```python
from build123d import *

# Parameters (mm, degrees)
SKETCH_1_W          = 15
SKETCH_1_H          = 15
SKETCH_1_W_2        = 13
SKETCH_1_H_2        = 13
EXTRUDE_1_DEPTH     = 125
CUT_EXTRUDE_1_REACH = 128.12
SKETCH_2_R          = 1.575
CUT_EXTRUDE_2_REACH = 128.12
SKETCH_3_R          = 1.6


with BuildPart() as part:
    # 草图1 → 凸台-拉伸1 (new body)
    with BuildSketch(Plane(origin=(0, 0, 0), x_dir=(1, 0, 0), z_dir=(0, 1, 0))):
        Rectangle(SKETCH_1_W, SKETCH_1_H)
        Rectangle(SKETCH_1_W_2, SKETCH_1_H_2, mode=Mode.SUBTRACT)
    extrude(amount=EXTRUDE_1_DEPTH)

    # 切除-拉伸1: up to this face of the body (flat: up to its plane)
    cut_extrude_1_end = Plane(part.part.faces().sort_by_distance((0, 62.5, -7.5))[0])
    # 草图2 → 切除-拉伸1 (cut, up to the picked face)
    with BuildSketch(Plane.XY.offset(7.5), mode=Mode.PRIVATE) as cut_extrude_1_sk1:
        with Locations((-3.75, 67.5)):
            Circle(SKETCH_2_R)
    cut_extrude_1_tool1 = split(extrude(cut_extrude_1_sk1.sketch, amount=-CUT_EXTRUDE_1_REACH, mode=Mode.PRIVATE), bisect_by=cut_extrude_1_end, keep=Keep.BOTH, mode=Mode.PRIVATE)
    # 草图2 → 切除-拉伸1 (cut, up to the picked face)
    with BuildSketch(Plane.XY.offset(7.5), mode=Mode.PRIVATE) as cut_extrude_1_sk2:
        with Locations((3.75, 67.5)):
            Circle(SKETCH_2_R)
    cut_extrude_1_tool2 = split(extrude(cut_extrude_1_sk2.sketch, amount=-CUT_EXTRUDE_1_REACH, mode=Mode.PRIVATE), bisect_by=cut_extrude_1_end, keep=Keep.BOTH, mode=Mode.PRIVATE)
    # 草图2 → 切除-拉伸1 (cut, up to the picked face)
    with BuildSketch(Plane.XY.offset(7.5), mode=Mode.PRIVATE) as cut_extrude_1_sk3:
        with Locations((-3.75, 57.5)):
            Circle(SKETCH_2_R)
    cut_extrude_1_tool3 = split(extrude(cut_extrude_1_sk3.sketch, amount=-CUT_EXTRUDE_1_REACH, mode=Mode.PRIVATE), bisect_by=cut_extrude_1_end, keep=Keep.BOTH, mode=Mode.PRIVATE)
    # 草图2 → 切除-拉伸1 (cut, up to the picked face)
    with BuildSketch(Plane.XY.offset(7.5), mode=Mode.PRIVATE) as cut_extrude_1_sk4:
        with Locations((3.75, 57.5)):
            Circle(SKETCH_2_R)
    cut_extrude_1_tool4 = split(extrude(cut_extrude_1_sk4.sketch, amount=-CUT_EXTRUDE_1_REACH, mode=Mode.PRIVATE), bisect_by=cut_extrude_1_end, keep=Keep.BOTH, mode=Mode.PRIVATE)
    # 草图2 → 切除-拉伸1 (cut, up to the picked face)
    with BuildSketch(Plane.XY.offset(7.5), mode=Mode.PRIVATE) as cut_extrude_1_sk5:
        with Locations((3.75, 120)):
            Circle(SKETCH_2_R)
    cut_extrude_1_tool5 = split(extrude(cut_extrude_1_sk5.sketch, amount=-CUT_EXTRUDE_1_REACH, mode=Mode.PRIVATE), bisect_by=cut_extrude_1_end, keep=Keep.BOTH, mode=Mode.PRIVATE)
    # 草图2 → 切除-拉伸1 (cut, up to the picked face)
    with BuildSketch(Plane.XY.offset(7.5), mode=Mode.PRIVATE) as cut_extrude_1_sk6:
        with Locations((-3.75, 120)):
            Circle(SKETCH_2_R)
    cut_extrude_1_tool6 = split(extrude(cut_extrude_1_sk6.sketch, amount=-CUT_EXTRUDE_1_REACH, mode=Mode.PRIVATE), bisect_by=cut_extrude_1_end, keep=Keep.BOTH, mode=Mode.PRIVATE)
    # 草图2 → 切除-拉伸1 (cut, up to the picked face)
    with BuildSketch(Plane.XY.offset(7.5), mode=Mode.PRIVATE) as cut_extrude_1_sk7:
        with Locations((-3.75, 110)):
            Circle(SKETCH_2_R)
    cut_extrude_1_tool7 = split(extrude(cut_extrude_1_sk7.sketch, amount=-CUT_EXTRUDE_1_REACH, mode=Mode.PRIVATE), bisect_by=cut_extrude_1_end, keep=Keep.BOTH, mode=Mode.PRIVATE)
    # 草图2 → 切除-拉伸1 (cut, up to the picked face)
    with BuildSketch(Plane.XY.offset(7.5), mode=Mode.PRIVATE) as cut_extrude_1_sk8:
        with Locations((3.75, 110)):
            Circle(SKETCH_2_R)
    cut_extrude_1_tool8 = split(extrude(cut_extrude_1_sk8.sketch, amount=-CUT_EXTRUDE_1_REACH, mode=Mode.PRIVATE), bisect_by=cut_extrude_1_end, keep=Keep.BOTH, mode=Mode.PRIVATE)
    # 草图2 → 切除-拉伸1 (cut, up to the picked face)
    with BuildSketch(Plane.XY.offset(7.5), mode=Mode.PRIVATE) as cut_extrude_1_sk9:
        with Locations((3.75, 15)):
            Circle(SKETCH_2_R)
    cut_extrude_1_tool9 = split(extrude(cut_extrude_1_sk9.sketch, amount=-CUT_EXTRUDE_1_REACH, mode=Mode.PRIVATE), bisect_by=cut_extrude_1_end, keep=Keep.BOTH, mode=Mode.PRIVATE)
    # 草图2 → 切除-拉伸1 (cut, up to the picked face)
    with BuildSketch(Plane.XY.offset(7.5), mode=Mode.PRIVATE) as cut_extrude_1_sk10:
        with Locations((-3.75, 15)):
            Circle(SKETCH_2_R)
    cut_extrude_1_tool10 = split(extrude(cut_extrude_1_sk10.sketch, amount=-CUT_EXTRUDE_1_REACH, mode=Mode.PRIVATE), bisect_by=cut_extrude_1_end, keep=Keep.BOTH, mode=Mode.PRIVATE)
    # 草图2 → 切除-拉伸1 (cut, up to the picked face)
    with BuildSketch(Plane.XY.offset(7.5), mode=Mode.PRIVATE) as cut_extrude_1_sk11:
        with Locations((-3.75, 5)):
            Circle(SKETCH_2_R)
    cut_extrude_1_tool11 = split(extrude(cut_extrude_1_sk11.sketch, amount=-CUT_EXTRUDE_1_REACH, mode=Mode.PRIVATE), bisect_by=cut_extrude_1_end, keep=Keep.BOTH, mode=Mode.PRIVATE)
    # 草图2 → 切除-拉伸1 (cut, up to the picked face)
    with BuildSketch(Plane.XY.offset(7.5), mode=Mode.PRIVATE) as cut_extrude_1_sk12:
        with Locations((3.75, 5)):
            Circle(SKETCH_2_R)
    cut_extrude_1_tool12 = split(extrude(cut_extrude_1_sk12.sketch, amount=-CUT_EXTRUDE_1_REACH, mode=Mode.PRIVATE), bisect_by=cut_extrude_1_end, keep=Keep.BOTH, mode=Mode.PRIVATE)
    add(cut_extrude_1_tool1.solids().sort_by(Axis((-3.75, 67.5, 7.5), (0, 0, -1)))[0], mode=Mode.SUBTRACT)
    add(cut_extrude_1_tool2.solids().sort_by(Axis((3.75, 67.5, 7.5), (0, 0, -1)))[0], mode=Mode.SUBTRACT)
    add(cut_extrude_1_tool3.solids().sort_by(Axis((-3.75, 57.5, 7.5), (0, 0, -1)))[0], mode=Mode.SUBTRACT)
    add(cut_extrude_1_tool4.solids().sort_by(Axis((3.75, 57.5, 7.5), (0, 0, -1)))[0], mode=Mode.SUBTRACT)
    add(cut_extrude_1_tool5.solids().sort_by(Axis((3.75, 120, 7.5), (0, 0, -1)))[0], mode=Mode.SUBTRACT)
    add(cut_extrude_1_tool6.solids().sort_by(Axis((-3.75, 120, 7.5), (0, 0, -1)))[0], mode=Mode.SUBTRACT)
    add(cut_extrude_1_tool7.solids().sort_by(Axis((-3.75, 110, 7.5), (0, 0, -1)))[0], mode=Mode.SUBTRACT)
    add(cut_extrude_1_tool8.solids().sort_by(Axis((3.75, 110, 7.5), (0, 0, -1)))[0], mode=Mode.SUBTRACT)
    add(cut_extrude_1_tool9.solids().sort_by(Axis((3.75, 15, 7.5), (0, 0, -1)))[0], mode=Mode.SUBTRACT)
    add(cut_extrude_1_tool10.solids().sort_by(Axis((-3.75, 15, 7.5), (0, 0, -1)))[0], mode=Mode.SUBTRACT)
    add(cut_extrude_1_tool11.solids().sort_by(Axis((-3.75, 5, 7.5), (0, 0, -1)))[0], mode=Mode.SUBTRACT)
    add(cut_extrude_1_tool12.solids().sort_by(Axis((3.75, 5, 7.5), (0, 0, -1)))[0], mode=Mode.SUBTRACT)

    # 切除-拉伸2: up to this face of the body (flat: up to its plane)
    cut_extrude_2_end = Plane(part.part.faces().sort_by_distance((7.5, 62.5, 0))[0])
    # 草图3 → 切除-拉伸2 (cut, up to the picked face)
    with BuildSketch(Plane.ZY.offset(7.5), mode=Mode.PRIVATE) as cut_extrude_2_sk1:
        with Locations((-3.75, 87.5)):
            Circle(SKETCH_3_R)
    cut_extrude_2_tool1 = split(extrude(cut_extrude_2_sk1.sketch, amount=-CUT_EXTRUDE_2_REACH, mode=Mode.PRIVATE), bisect_by=cut_extrude_2_end, keep=Keep.BOTH, mode=Mode.PRIVATE)
    # 草图3 → 切除-拉伸2 (cut, up to the picked face)
    with BuildSketch(Plane.ZY.offset(7.5), mode=Mode.PRIVATE) as cut_extrude_2_sk2:
        with Locations((3.75, 87.5)):
            Circle(SKETCH_3_R)
    cut_extrude_2_tool2 = split(extrude(cut_extrude_2_sk2.sketch, amount=-CUT_EXTRUDE_2_REACH, mode=Mode.PRIVATE), bisect_by=cut_extrude_2_end, keep=Keep.BOTH, mode=Mode.PRIVATE)
    # 草图3 → 切除-拉伸2 (cut, up to the picked face)
    with BuildSketch(Plane.ZY.offset(7.5), mode=Mode.PRIVATE) as cut_extrude_2_sk3:
        with Locations((-3.75, 77.5)):
            Circle(SKETCH_3_R)
    cut_extrude_2_tool3 = split(extrude(cut_extrude_2_sk3.sketch, amount=-CUT_EXTRUDE_2_REACH, mode=Mode.PRIVATE), bisect_by=cut_extrude_2_end, keep=Keep.BOTH, mode=Mode.PRIVATE)
    # 草图3 → 切除-拉伸2 (cut, up to the picked face)
    with BuildSketch(Plane.ZY.offset(7.5), mode=Mode.PRIVATE) as cut_extrude_2_sk4:
        with Locations((3.75, 77.5)):
            Circle(SKETCH_3_R)
    cut_extrude_2_tool4 = split(extrude(cut_extrude_2_sk4.sketch, amount=-CUT_EXTRUDE_2_REACH, mode=Mode.PRIVATE), bisect_by=cut_extrude_2_end, keep=Keep.BOTH, mode=Mode.PRIVATE)
    # 草图3 → 切除-拉伸2 (cut, up to the picked face)
    with BuildSketch(Plane.ZY.offset(7.5), mode=Mode.PRIVATE) as cut_extrude_2_sk5:
        with Locations((3.75, 47.5)):
            Circle(SKETCH_3_R)
    cut_extrude_2_tool5 = split(extrude(cut_extrude_2_sk5.sketch, amount=-CUT_EXTRUDE_2_REACH, mode=Mode.PRIVATE), bisect_by=cut_extrude_2_end, keep=Keep.BOTH, mode=Mode.PRIVATE)
    # 草图3 → 切除-拉伸2 (cut, up to the picked face)
    with BuildSketch(Plane.ZY.offset(7.5), mode=Mode.PRIVATE) as cut_extrude_2_sk6:
        with Locations((-3.75, 47.5)):
            Circle(SKETCH_3_R)
    cut_extrude_2_tool6 = split(extrude(cut_extrude_2_sk6.sketch, amount=-CUT_EXTRUDE_2_REACH, mode=Mode.PRIVATE), bisect_by=cut_extrude_2_end, keep=Keep.BOTH, mode=Mode.PRIVATE)
    # 草图3 → 切除-拉伸2 (cut, up to the picked face)
    with BuildSketch(Plane.ZY.offset(7.5), mode=Mode.PRIVATE) as cut_extrude_2_sk7:
        with Locations((3.75, 37.5)):
            Circle(SKETCH_3_R)
    cut_extrude_2_tool7 = split(extrude(cut_extrude_2_sk7.sketch, amount=-CUT_EXTRUDE_2_REACH, mode=Mode.PRIVATE), bisect_by=cut_extrude_2_end, keep=Keep.BOTH, mode=Mode.PRIVATE)
    # 草图3 → 切除-拉伸2 (cut, up to the picked face)
    with BuildSketch(Plane.ZY.offset(7.5), mode=Mode.PRIVATE) as cut_extrude_2_sk8:
        with Locations((-3.75, 37.5)):
            Circle(SKETCH_3_R)
    cut_extrude_2_tool8 = split(extrude(cut_extrude_2_sk8.sketch, amount=-CUT_EXTRUDE_2_REACH, mode=Mode.PRIVATE), bisect_by=cut_extrude_2_end, keep=Keep.BOTH, mode=Mode.PRIVATE)
    add(cut_extrude_2_tool1.solids().sort_by(Axis((-7.5, 87.5, -3.75), (1, 0, 0)))[0], mode=Mode.SUBTRACT)
    add(cut_extrude_2_tool2.solids().sort_by(Axis((-7.5, 87.5, 3.75), (1, 0, 0)))[0], mode=Mode.SUBTRACT)
    add(cut_extrude_2_tool3.solids().sort_by(Axis((-7.5, 77.5, -3.75), (1, 0, 0)))[0], mode=Mode.SUBTRACT)
    add(cut_extrude_2_tool4.solids().sort_by(Axis((-7.5, 77.5, 3.75), (1, 0, 0)))[0], mode=Mode.SUBTRACT)
    add(cut_extrude_2_tool5.solids().sort_by(Axis((-7.5, 47.5, 3.75), (1, 0, 0)))[0], mode=Mode.SUBTRACT)
    add(cut_extrude_2_tool6.solids().sort_by(Axis((-7.5, 47.5, -3.75), (1, 0, 0)))[0], mode=Mode.SUBTRACT)
    add(cut_extrude_2_tool7.solids().sort_by(Axis((-7.5, 37.5, 3.75), (1, 0, 0)))[0], mode=Mode.SUBTRACT)
    add(cut_extrude_2_tool8.solids().sort_by(Axis((-7.5, 37.5, -3.75), (1, 0, 0)))[0], mode=Mode.SUBTRACT)


solid = part.part
```
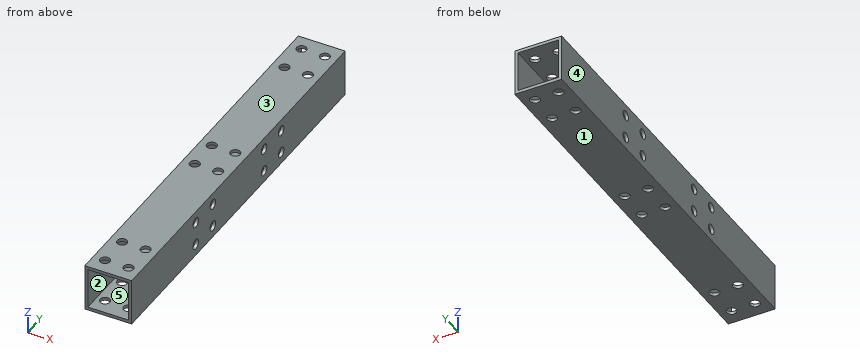
CAD build for the part. Positions are in the model's coordinates, mm. Face numbers are marked on the shaded views. A direction names the side the tool comes from. Give positions to 0.01 mm unless a question says otherwise; leave off trailing zeros. Loops run counter-clockwise (first coordinate to the right, second up) from the corner with the lowest first, then second, coordinate; pieces in that order, holes last. Notation, with made-up numbers: (-12.75, 34) - (-2.75, 34) arc R17 cw to (-2.75, 44) - close; hole circle Ø11 at (40, -10). An arc over 180 degrees is marked (long way). Put each result on its own line as item: value.
Q1. Flat gauge pin, fed straight in: pin 1 (2.5 mm diameter, centred on y = 87.5, z = 3.75, fed in from -X). Where does the tip first touch, or does it go through?
Filled in:
pin 1: passes through
Q2. Tool access for the marked faces 1 and 2: list every direction of +Z, -Z, +X, -X, +Y, -Y with a clear straight run to the whole face (end or side of a thin tool).
Filled in:
face 1: -Z, +X, -X, +Y, -Y
face 2: +Y, -Y
Q3. Slice it at D-D (x = -3.75). Give the number of separate pieces and of enclosed holes in the cut face, plus the area to 3 significant figures.
Filled in:
separate pieces: 14
enclosed holes: 0
area: 212 mm²
Q4. Slice it at C-C (y = 15). Give the cut face in (x, z) (3 decimals), plus the area to 3 significant figures.
Filled in:
outline: (-7.5, -7.5) - (-5.325, -7.5) - (-5.325, -6.5) - (-6.5, -6.5) - (-6.5, 6.5) - (-5.325, 6.5) - (-5.325, 7.5) - (-7.5, 7.5) - close; (-2.175, -7.5) - (2.175, -7.5) - (2.175, -6.5) - (-2.175, -6.5) - close; (-2.175, 6.5) - (2.175, 6.5) - (2.175, 7.5) - (-2.175, 7.5) - close; (5.325, -7.5) - (7.5, -7.5) - (7.5, 7.5) - (5.325, 7.5) - (5.325, 6.5) - (6.5, 6.5) - (6.5, -6.5) - (5.325, -6.5) - close
area: 43.4 mm²
Q5. Mould opens along X. For the marked faces 3, 4 and 5 say: pulls with the +X half, pulls with the -X half, needs draft (parallel to the pull), parting line crosses it, or undercut.
Filled in:
face 3: needs draft
face 4: pulls with the -X half
face 5: undercut
Q6. Slice it at B-B (z = 1). Give the cut face in (x, y).
Filled in:
outline: (-7.5, 0) - (-6.5, 0) - (-6.5, 125) - (-7.5, 125) - close; (6.5, 0) - (7.5, 0) - (7.5, 125) - (6.5, 125) - close
Q7. Slice it at A-A (y = 52). Give the cut face in (x, z).
Filled in:
outline: (-7.5, -7.5) - (7.5, -7.5) - (7.5, 7.5) - (-7.5, 7.5) - close; hole (-6.5, -6.5) - (6.5, -6.5) - (6.5, 6.5) - (-6.5, 6.5) - close
Q8. Probe line 1 along Y through (x, z) = (-6.8, -3.75); line 2 along Z through (x, y) = (-6.85, 87.5); line 3 along X through (y, z) = (120, -7.2) (3 decimals). List the from-to ranges inside material, lowest first.
Filled in:
line 1: y = 0 to 35.9, 39.1 to 45.9, 49.1 to 75.9, 79.1 to 85.9, 89.1 to 125
line 2: z = -7.5 to -5.35, -2.15 to 2.15, 5.35 to 7.5
line 3: x = -7.5 to -5.325, -2.175 to 2.175, 5.325 to 7.5
